```python
from build123d import *

# Parameters (mm, degrees)
ESQUISSE1_R             = 11
BOSS_EXTRU_1_DEPTH      = 5
BOSS_EXTRU_3_DEPTH      = 5
CONG_3_R                = 0.5
ESQUISSE3D1_R           = 1.05
ENL_V_MAT_EXTRU_1_DEPTH = 25.164275332
ESQUISSE3D2_R           = 1.75
ENL_V_MAT_EXTRU_2_DEPTH = 2.5
ESQUISSE4_R             = 1.75
ENL_V_MAT_EXTRU_3_DEPTH = 17.340134669


with BuildPart() as part:
    # Esquisse1 → Boss.-Extru.1 (new body)
    with BuildSketch(Plane.XY):
        Circle(ESQUISSE1_R)
    extrude(amount=BOSS_EXTRU_1_DEPTH)

    # Esquisse2 → Boss.-Extru.3 (add)
    with BuildSketch(Plane.XY.offset(5)):
        with BuildLine():
            ThreePointArc((-2.5, 10.712142643), (-4.878752687, 9.858893053), (-7, 8.485281374))
            Line((-7, 8.485281374), (-7, -8.485281374))
            ThreePointArc((-7, -8.485281374), (-4.878752687, -9.858893053), (-2.5, -10.712142643))
            Line((-2.5, -10.712142643), (-2.5, 10.712142643))
        make_face()
        with BuildLine():
            ThreePointArc((7, 8.485281374), (4.878752687, 9.858893053), (2.5, 10.712142643))
            Line((2.5, 10.712142643), (2.5, -10.712142643))
            ThreePointArc((2.5, -10.712142643), (4.878752687, -9.858893053), (7, -8.485281374))
            Line((7, -8.485281374), (7, 8.485281374))
        make_face()
    extrude(amount=BOSS_EXTRU_3_DEPTH)

    # Congé3
    cong_3_edges = [part.edges().sort_by_distance(p)[0] for p in [
        (4.878752687, 9.858893053, 10),
        (4.878752687, -9.858893053, 10),
        (7, 0, 10),
        (2.5, 0, 10),
        (-4.878752687, 9.858893053, 10),
        (-4.878752687, -9.858893053, 10),
        (-2.5, 0, 10),
        (-7, 0, 10),
    ]]
    fillet(cong_3_edges, radius=CONG_3_R)

    # Esquisse3D1 → Enlèv. mat.-Extru.1 (cut, through all)
    with BuildSketch(Plane(origin=(0.000157277, -8.050163785, 0), x_dir=(0, 1, 0), z_dir=(0, 0, -1))):
        with Locations(Location((0, 0, 0), (0, 0, 90))):
            Circle(ESQUISSE3D1_R)
        with Locations(Location((8, 8, 0), (0, 0, 90))):
            Circle(ESQUISSE3D1_R)
        with Locations(Location((16, 0, 0), (0, 0, 90))):
            Circle(ESQUISSE3D1_R)
        with Locations(Location((8, -8, 0), (0, 0, 90))):
            Circle(ESQUISSE3D1_R)
    extrude(amount=-ENL_V_MAT_EXTRU_1_DEPTH, mode=Mode.SUBTRACT)

    # Esquisse3D2 → Enlèv. mat.-Extru.2 (cut)
    with BuildSketch(Plane(origin=(-8, 0, 5), x_dir=(0.9999950851821525, -0.0031352211308848022, 0), z_dir=(0, 0, 1))):
        with Locations(Location((0, 0, 0), (0, 0, 305.029539812))):
            Circle(ESQUISSE3D2_R)
        with Locations(Location((8.075049898, -7.974722127, 0), (0, 0, 0.179635233))):
            Circle(ESQUISSE3D2_R)
        with Locations(Location((7.974878912, 8.025042451, 0), (0, 0, 0.179635233))):
            Circle(ESQUISSE3D2_R)
        with Locations(Location((16.000078637, 0, 0), (0, 0, 235.329730654))):
            Circle(ESQUISSE3D2_R)
    extrude(amount=-ENL_V_MAT_EXTRU_2_DEPTH, mode=Mode.SUBTRACT)

    # Esquisse4 → Enlèv. mat.-Extru.3 (cut, through all)
    with BuildSketch(Plane.XY.offset(5)):
        with Locations((-7.999842723, -0.050163785)):
            Circle(ESQUISSE4_R)
        with Locations((8.000157277, -0.050163785)):
            Circle(ESQUISSE4_R)
    extrude(amount=ENL_V_MAT_EXTRU_3_DEPTH, mode=Mode.SUBTRACT)


solid = part.part
```
Could you check a few things on this model? Use its own coordinates, in mm. A direction names the side the tool comes from. Round coordinates to 2 decimals unless told otherwise and drop trailing zeros. Loops run counter-clockwise (first coordinate to the right, second up) from the corner with the lowest first, then second, coordinate; pieces in that order, holes last. Notation, with made-up numbers: (63, 37.5) - (118, 37.5) arc R21 ccw to (118, 49.5) - close; hole circle Ø10 at (34, -34). An arc over 180 degrees is marked (long way). Answer in a Markdown table with one row per item. Add a question column.
(1) If we section it at A-A (z = 8): Please give me the cut outline in (x, y), plus the area to 3 significant figures.
(2) If we mould it in two halves opening along X, with no side actions, what happens to faces 1 (the face through (-5, 0, 10)), 2 (the face through (7, 5, 7)), 3 (the face through (-1, 7, 2.5))? For each: pulls with the +X half, pulls with the -X half, needs draft (parallel to the pull), parting line crosses it, or undercut.
(3) I'm going to push flat-ended pins straight in: pin 1 (1 mm diameter, centred on x = 5.5, y = 6.5, fed in from -Z); pin 2 (1.3 mm diameter, centred on y = 3, z = 7, fed in from +X); pin 3 (3 mm diameter, centred on y = 4.5, z = 1.5, fed in from +X); pin 4 (1.7 mm diameter, centred on x = 0, y = -8.05, fed in from -Z). Where does each tip first touch, or does it pass through?
(4) If we section it at D-D (y = 5.25): Please give me the cut outline in (x, z).
(5) For faces 4 (the face through (-6.25, -0.07, 7.47)), 5 (the face through (-0.228, 9.735, 3.768)), 6 (the face through (0, 0, 5)), which set-ups out of +Z, -Z, +X, -X, +Y, -Y let a thin tool reach every point of the face, with its end or its side?
(6) If we section it at B-B (y = -0.5): State how many separate pieces and enclosed holes the cut face has, plus the area to 3 significant figures.
(7) If we section it at C-C (x = 8): Please give me the cut outline in (y, z), plus the area to 3 significant figures.
(8) I need wall thicknesses on line 1 along X through (y, z) = (0, 4.05); line 2 along X through (y, z) = (6.5, 8.25). Which ranges of each line are inside material? Lowest first, please.
Model answer:
| question | item | result |
|---|---|---|
| 1 | outline | (-7, -8.49) arc R11 ccw to (-2.5, -10.71) - (-2.5, 10.71) arc R11 ccw to (-7, 8.49) - (-7, 1.39) arc R1.75 cw to (-7, -1.49) - close; (2.5, -10.71) arc R11 ccw to (7, -8.49) - (7, -1.49) arc R1.75 cw to (7, 1.39) - (7, 8.49) arc R11 ccw to (2.5, 10.71) - close |
| 1 | area | 174 mm² |
| 2 | face 1 | needs draft |
| 2 | face 2 | pulls with the +X half |
| 2 | face 3 | undercut |
| 3 | pin 1 | stops at z = 0 |
| 3 | pin 2 | stops at x = 7 |
| 3 | pin 3 | stops at x = 10.58 |
| 3 | pin 4 | passes through |
| 4 | outline | (-9.67, 0) - (9.67, 0) - (9.67, 5) - (7, 5) - (7, 9.5) arc R0.5 ccw to (6.5, 10) - (3, 10) arc R0.5 ccw to (2.5, 9.5) - (2.5, 5) - (-2.5, 5) - (-2.5, 9.5) arc R0.5 ccw to (-3, 10) - (-6.5, 10) arc R0.5 ccw to (-7, 9.5) - (-7, 5) - (-9.67, 5) - close |
| 5 | face 4 | +Z, -X |
| 5 | face 5 | +Z |
| 5 | face 6 | +Z, +Y, -Y |
| 6 | separate pieces | 3 |
| 6 | enclosed holes | 0 |
| 6 | area | 122 mm² |
| 7 | outline | (-7.55, 0) - (-1.1, 0) - (-1.1, 2.5) - (-1.8, 2.5) - (-1.8, 5) - (-7.55, 5) - close; (1, 0) - (7.55, 0) - (7.55, 5) - (1.7, 5) - (1.7, 2.5) - (1, 2.5) - close |
| 7 | area | 61.5 mm² |
| 8 | line 1 | x = -11 to -9.75, -6.25 to 6.25, 9.75 to 11 |
| 8 | line 2 | x = -7 to -2.5, 2.5 to 7 |
